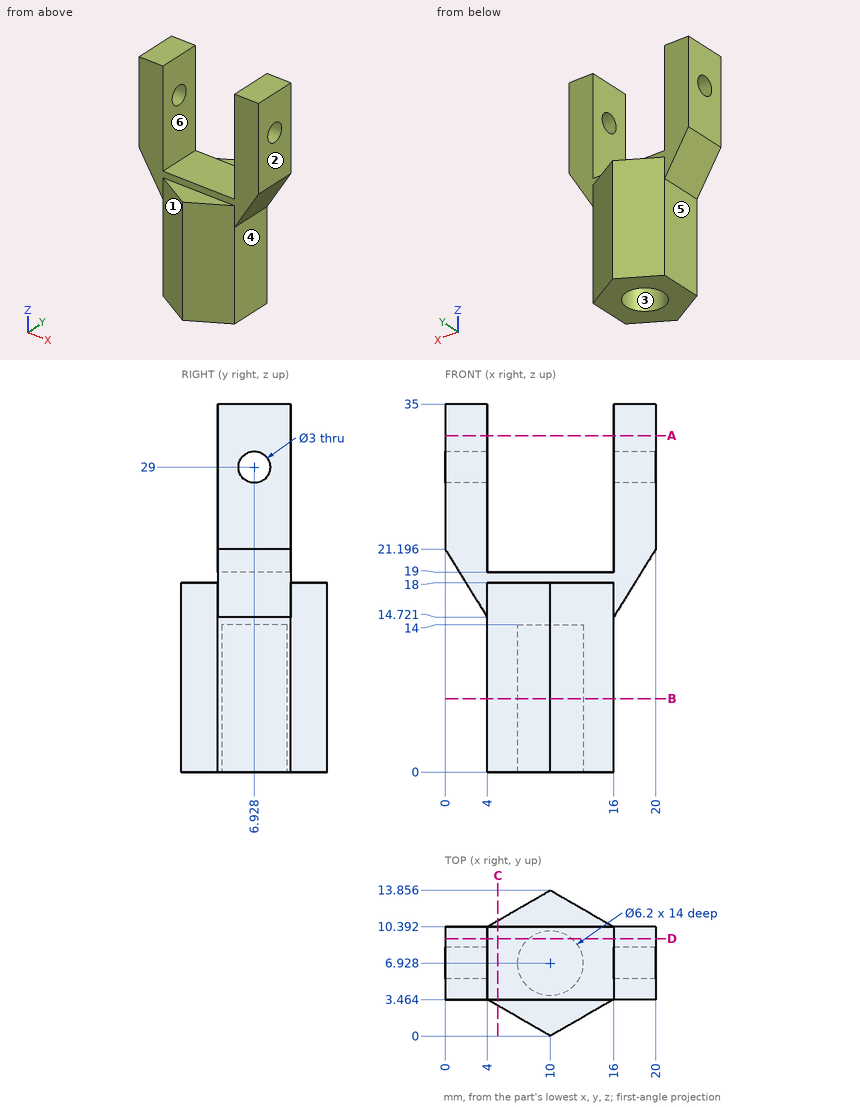
Design review of the part shown in the three views and the two pictorial views. Dimensions are in mm from the part's minimum x, y and z. A direction names the side the tool comes from. Give positions to 0.01 mm unless a question says otherwise; leave off trailing zeros. Write each loop counter-clockwise with the first axis right and the second up, starting at its lowest first coordinate (ties: lowest second). Pieces come first, ordered by that corner, then holes. Notation, with made-up numbers: M 43.25,-35.5 L 79.25,-35.5 A25 ccw 79.25,2.5 Z; hole C -30,81 d7. An arc over 180 degrees is marked long. Return JSON: item names as keys, results as strings. Group by question number.
Item 1: Take a section at A-A (z = 32). Give the boundary of the cut face in (x, y).
Item 2: Take a section at C-C (x = 5). Give the boundary of the cut face in (y, z).
Item 3: Wall thickness on line 1 along X through (y, z) = (8.75, 25); line 2 along Y through (x, z) = (18.95, 29); line 3 along Z through (x, y) = (6, 5.5): over which ranges is each line inside the solid? List them lowest first.
Item 4: Take a section at D-D (y = 9.25). Give the boundary of the cut face in (x, z) (1 decimal).
Item 5: Tool access review of the marked faces 4, 5 and 6: name each direction out of +Z, -Z, +X, -X, +Y, -Y from which nothing blocks a thin tool from reaching the whole face with its end or side.
Item 6: Clearance check with flat-ended pins moving along their axes: pin 1 Ø3.5 at (y, z) = (6.93, 29) entering from +X; pin 2 Ø6 at (x, z) = (14.5, 22) entering from -Y; pin 3 Ø3.5 at (x, y) = (10, 6.93) entering from -Z; pin 4 Ø4 at (x, y) = (12, 11.5) entering from +Z. State where each tip first meets the part, or that it passes through.
Item 7: The part is to be moulded in two halves that separate along Y. For the marked faces 1, 2 and 3, say which applies: pulls with the +Y half, pulls with the -Y half, needs draft (parallel to the pull), parting line crosses it, or undercut.
Item 8: Take a section at B-B (z = 7). Give the boundary of the cut face in (x, y).
Return value:
{
 "1": {"outline": "M 0,3.46 L 4,3.46 L 4,10.39 L 0,10.39 Z; M 16,3.46 L 20,3.46 L 20,10.39 L 16,10.39 Z"},
 "2": {"outline": "M 2.89,0 L 10.97,0 L 10.97,18 L 10.39,18 L 10.39,19 L 3.46,19 L 3.46,18 L 2.89,18 Z"},
 "3": {"line 1": "x = 0 to 4, 16 to 20", "line 2": "y = 3.46 to 5.43, 8.43 to 10.39", "line 3": "z = 0 to 19"},
 "4": {"outline": "M 0,21.2 L 4,14.7 L 4,0 L 7.9,0 L 7.9,14 L 12.1,14 L 12.1,0 L 16,0 L 16,14.7 L 20,21.2 L 20,35 L 16,35 L 16,19 L 4,19 L 4,35 L 0,35 Z"},
 "5": {"face 4": "-Z, +X, +Y, -Y", "face 5": "-Z, -X, +Y, -Y", "face 6": "+Z, +Y, -Y"},
 "6": {"pin 1": "stops at x = 20", "pin 2": "stops at y = 3.46", "pin 3": "stops at z = 14", "pin 4": "stops at z = 19"},
 "7": {"face 1": "pulls with the -Y half", "face 2": "needs draft", "face 3": "undercut"},
 "8": {"outline": "M 4,3.46 L 10,0 L 16,3.46 L 16,10.39 L 10,13.86 L 4,10.39 Z; hole C 10,6.93 d6.2"}
}
